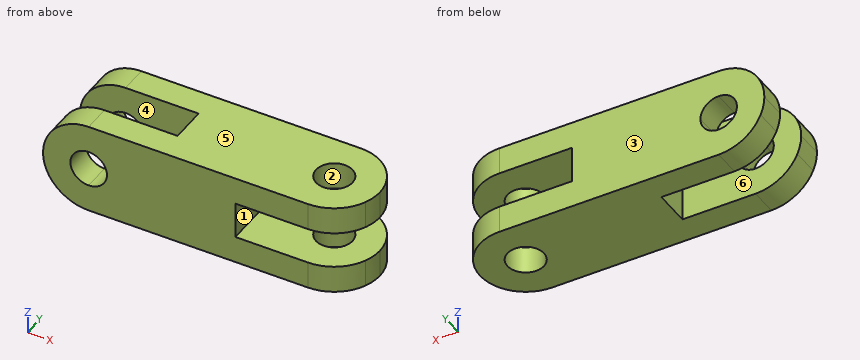
from build123d import *

# Parameters (mm, degrees)
F0_R     = 6.35
F1_DEPTH = 31.75
F0_W     = 41.275
F0_H     = 12.7
F3_DEPTH = 31.75
F2_W     = 41.275
F2_H     = 12.7
F4_DEPTH = 31.751
F5_DEPTH = 31.751


with BuildPart() as f1:
    # F0 (on Top) → F1 (new body)
    with BuildSketch(Plane.XY):
        with BuildLine():
            ThreePointArc((35.5833037704, -18.7424994532), (22.3013258492, -11.5625950536), (21.0336259389, 3.4825005468))
            Line((21.0336259389, 3.4825005468), (-15.2166962296, 3.4825005468))
            Line((-15.2166962296, 3.4825005468), (-15.2166962296, -9.2174994532))
            Line((-15.2166962296, -9.2174994532), (-56.4916962296, -9.2174994532))
            Line((-56.4916962296, -9.2174994532), (-56.4916962296, -18.7424994532))
            Line((-56.4916962296, -18.7424994532), (35.5833037704, -18.7424994532))
        make_face()
        with BuildLine():
            Line((35.5833037704, 13.0075005468), (-56.4916962296, 13.0075005468))
            Line((-56.4916962296, 13.0075005468), (-56.4916962296, 3.4825005468))
            Line((-56.4916962296, 3.4825005468), (-15.2166962296, 3.4825005468))
            Line((-15.2166962296, 3.4825005468), (21.0336259389, 3.4825005468))
            ThreePointArc((21.0336259389, 3.4825005468), (26.88820817, 10.414478468), (35.5833037704, 13.0075005468))
        make_face()
        with BuildLine():
            ThreePointArc((50.1329816019, 3.4825005468), (44.2783993708, 10.414478468), (35.5833037704, 13.0075005468))
            ThreePointArc((35.5833037704, 13.0075005468), (26.88820817, 10.414478468), (21.0336259389, 3.4825005468))
            ThreePointArc((21.0336259389, 3.4825005468), (22.3013258492, -11.5625950536), (35.5833037704, -18.7424994532))
            ThreePointArc((35.5833037704, -18.7424994532), (44.2783993708, -16.1494773745), (50.1329816019, -9.2174994532))
            ThreePointArc((50.1329816019, -9.2174994532), (51.1234414882, -6.1109150468), (51.4583037704, -2.8674994532))
            ThreePointArc((51.4583037704, -2.8674994532), (51.1234414882, 0.3759161403), (50.1329816019, 3.4825005468))
        make_face()
        with Locations((35.5833037704, -2.8674994532)):
            Circle(F0_R, mode=Mode.SUBTRACT)
        with BuildLine():
            ThreePointArc((50.1329816019, -9.2174994532), (44.2783993708, -16.1494773745), (35.5833037704, -18.7424994532))
            Line((35.5833037704, -18.7424994532), (51.6392476857, -18.7424994532))
            Line((51.6392476857, -18.7424994532), (51.4583037704, -9.2174994532))
            Line((51.4583037704, -9.2174994532), (50.1329816019, -9.2174994532))
        make_face()
        with BuildLine():
            Line((51.2197911739, 13.0075005468), (35.5833037704, 13.0075005468))
            ThreePointArc((35.5833037704, 13.0075005468), (44.2783993708, 10.414478468), (50.1329816019, 3.4825005468))
            Line((50.1329816019, 3.4825005468), (51.4583037704, 3.4825005468))
            Line((51.4583037704, 3.4825005468), (51.2197911739, 13.0075005468))
        make_face()
    extrude(amount=F1_DEPTH)

    # F0 (on Top) → F3 (cut)
    with BuildSketch(Plane.XY):
        with BuildLine():
            Line((35.5833037704, 13.0075005468), (-56.4916962296, 13.0075005468))
            Line((-56.4916962296, 13.0075005468), (-56.4916962296, 3.4825005468))
            Line((-56.4916962296, 3.4825005468), (-15.2166962296, 3.4825005468))
            Line((-15.2166962296, 3.4825005468), (21.0336259389, 3.4825005468))
            ThreePointArc((21.0336259389, 3.4825005468), (26.88820817, 10.414478468), (35.5833037704, 13.0075005468))
        make_face()
        with BuildLine():
            Line((51.2197911739, 13.0075005468), (35.5833037704, 13.0075005468))
            ThreePointArc((35.5833037704, 13.0075005468), (44.2783993708, 10.414478468), (50.1329816019, 3.4825005468))
            Line((50.1329816019, 3.4825005468), (51.4583037704, 3.4825005468))
            Line((51.4583037704, 3.4825005468), (51.2197911739, 13.0075005468))
        make_face()
        with BuildLine():
            ThreePointArc((50.1329816019, 3.4825005468), (44.2783993708, 10.414478468), (35.5833037704, 13.0075005468))
            ThreePointArc((35.5833037704, 13.0075005468), (26.88820817, 10.414478468), (21.0336259389, 3.4825005468))
            ThreePointArc((21.0336259389, 3.4825005468), (22.3013258492, -11.5625950536), (35.5833037704, -18.7424994532))
            ThreePointArc((35.5833037704, -18.7424994532), (44.2783993708, -16.1494773745), (50.1329816019, -9.2174994532))
            ThreePointArc((50.1329816019, -9.2174994532), (51.1234414882, -6.1109150468), (51.4583037704, -2.8674994532))
            ThreePointArc((51.4583037704, -2.8674994532), (51.1234414882, 0.3759161403), (50.1329816019, 3.4825005468))
        make_face()
        with Locations((35.5833037704, -2.8674994532)):
            Circle(F0_R, mode=Mode.SUBTRACT)
        with Locations((-35.8541962296, -2.8674994532)):
            Rectangle(F0_W, F0_H)
        with BuildLine():
            ThreePointArc((35.5833037704, -18.7424994532), (22.3013258492, -11.5625950536), (21.0336259389, 3.4825005468))
            Line((21.0336259389, 3.4825005468), (-15.2166962296, 3.4825005468))
            Line((-15.2166962296, 3.4825005468), (-15.2166962296, -9.2174994532))
            Line((-15.2166962296, -9.2174994532), (-56.4916962296, -9.2174994532))
            Line((-56.4916962296, -9.2174994532), (-56.4916962296, -18.7424994532))
            Line((-56.4916962296, -18.7424994532), (35.5833037704, -18.7424994532))
        make_face()
        with BuildLine():
            ThreePointArc((50.1329816019, -9.2174994532), (44.2783993708, -16.1494773745), (35.5833037704, -18.7424994532))
            Line((35.5833037704, -18.7424994532), (51.6392476857, -18.7424994532))
            Line((51.6392476857, -18.7424994532), (51.4583037704, -9.2174994532))
            Line((51.4583037704, -9.2174994532), (50.1329816019, -9.2174994532))
        make_face()
    extrude(amount=-F3_DEPTH, mode=Mode.SUBTRACT)

    # F2 (on face) → F4 (cut, through all)
    with BuildSketch(Plane.XZ.offset(18.7424994532)):
        with BuildLine():
            Line((-56.4916962296, 31.75), (-56.4916962296, 22.225))
            Line((-56.4916962296, 22.225), (-55.1663740611, 22.225))
            ThreePointArc((-55.1663740611, 22.225), (-49.31179183, 29.1569779212), (-40.6166962296, 31.75))
            Line((-40.6166962296, 31.75), (-56.4916962296, 31.75))
        make_face()
        with BuildLine():
            Line((-55.1663740611, 22.225), (-56.4916962296, 22.225))
            Line((-56.4916962296, 22.225), (-56.4916962296, 15.875))
            ThreePointArc((-56.4916962296, 15.875), (-56.1568339474, 19.1184155936), (-55.1663740611, 22.225))
        make_face()
        with BuildLine():
            ThreePointArc((-55.1663740611, 9.525), (-56.1568339474, 12.6315844064), (-56.4916962296, 15.875))
            Line((-56.4916962296, 15.875), (-56.4916962296, 9.525))
            Line((-56.4916962296, 9.525), (-55.1663740611, 9.525))
        make_face()
        with BuildLine():
            ThreePointArc((-40.6166962296, 0), (-49.31179183, 2.5930220788), (-55.1663740611, 9.525))
            Line((-55.1663740611, 9.525), (-56.4916962296, 9.525))
            Line((-56.4916962296, 9.525), (-56.4916962296, 0))
            Line((-56.4916962296, 0), (-40.6166962296, 0))
        make_face()
        with BuildLine():
            Line((-40.6166962296, 9.525), (-40.6166962296, 22.225))
            ThreePointArc((-40.6166962296, 22.225), (-46.9666962296, 15.875), (-40.6166962296, 9.525))
        make_face()
        with BuildLine():
            ThreePointArc((-34.2666962296, 15.875), (-36.126568169, 20.3651280605), (-40.6166962296, 22.225))
            Line((-40.6166962296, 22.225), (-40.6166962296, 9.525))
            ThreePointArc((-40.6166962296, 9.525), (-36.126568169, 11.3848719395), (-34.2666962296, 15.875))
        make_face()
        with Locations((31.0017476857, 15.875)):
            Rectangle(F2_W, F2_H)
    extrude(amount=-F4_DEPTH, mode=Mode.SUBTRACT)

    # F0 (on Top) → F5 (cut, through all)
    with BuildSketch(Plane.XY):
        with BuildLine():
            Line((51.2197911739, 13.0075005468), (35.5833037704, 13.0075005468))
            ThreePointArc((35.5833037704, 13.0075005468), (44.2783993708, 10.414478468), (50.1329816019, 3.4825005468))
            Line((50.1329816019, 3.4825005468), (51.4583037704, 3.4825005468))
            Line((51.4583037704, 3.4825005468), (51.2197911739, 13.0075005468))
        make_face()
        with BuildLine():
            ThreePointArc((50.1329816019, -9.2174994532), (44.2783993708, -16.1494773745), (35.5833037704, -18.7424994532))
            Line((35.5833037704, -18.7424994532), (51.6392476857, -18.7424994532))
            Line((51.6392476857, -18.7424994532), (51.4583037704, -9.2174994532))
            Line((51.4583037704, -9.2174994532), (50.1329816019, -9.2174994532))
        make_face()
    extrude(amount=F5_DEPTH, mode=Mode.SUBTRACT)


solid = f1.part
Geometry check sheet. Reference: the model listing, model coordinates, mm. Face numbers are marked on the shaded views. A direction names the side the tool comes from. Round coordinates to 2 decimals unless told otherwise and drop trailing zeros. Order: outer loops, then holes, each group sorted by start corner. A loop starts at its lowest first (then second) coordinate and runs counter-clockwise, first axis right, second up. Notation, with made-up numbers: M 13.25,-40 L 67.25,-40 A14 cw 67.25,-22 Z; hole C -35,62 d11. An arc over 180 degrees is marked long. Answer in a Markdown table with one row per item.
(1) Tool access check on the marked faces 1 and 2. Record the directions out of +Z, -Z, +X, -X, +Y, -Y that give a thin tool (end or side, any length) a straight path to the whole face; none if there is none.
Responses:
| item | result |
|---|---|
| face 1 | +X, +Y, -Y |
| face 2 | +Z, -Z |
(2) Scan lines: probe 1 along Z at (x, y) = (32.5, 7.5) (3 decimals); probe 2 along Y at (x, z) = (-47, 25); probe 3 along X at (y, z) = (2, 16). Record each from-to range of solid material in increasing order. Write a range as from..to.
Responses:
| item | result |
|---|---|
| probe 1 | z = 0..9.525, 22.225..31.75 |
| probe 2 | y = -18.74..-9.22, 3.48..13.01 |
| probe 3 | x = -15.22..10.36 |
(3) Go/stop test with flat-tipped pins: P1, Ø3, axis at y = -15, z = 22, coming from the +X side; P2, Ø10, axis at y = -3, z = 16.5, coming from the +X side; P3, Ø10, axis at y = -3, z = 15.5, coming from the -X side; P4, Ø1.5, axis at x = 39, y = 1.5, coming from the +Z side (3 decimals). Record where each tip stops, or that it passes through.
Responses:
| item | result |
|---|---|
| P1 | stops at x = 47.36 |
| P2 | stops at x = 10.36 |
| P3 | stops at x = -15.22 |
| P4 | passes through |
(4) Sectioned sample at B-B, the plane z = 21. Record the cut outline in (x, y), and give its area (3 significant figures).
Responses:
| item | result |
|---|---|
| outline | M -55.64,-18.74 L -44.37,-18.74 L -44.37,-9.22 L -55.64,-9.22 Z; M -55.64,3.48 L -44.37,3.48 L -44.37,13.01 L -55.64,13.01 Z; M -36.87,-18.74 L 10.36,-18.74 L 10.36,13.01 L -36.87,13.01 L -36.87,3.48 L -15.22,3.48 L -15.22,-9.22 L -36.87,-9.22 Z |
| area | 1,440 mm² |
(5) Sectioned sample at C-C, the plane y = 0.5. Record the cut outline in (x, z) (3 decimals), and give its area (3 significant figures).
Responses:
| item | result |
|---|---|
| outline | M -15.217,0 L 30.2,0 L 30.2,9.525 L 10.364,9.525 L 10.364,22.225 L 30.2,22.225 L 30.2,31.75 L -15.217,31.75 Z; M 40.967,0 L 51.097,0 L 51.097,9.525 L 40.967,9.525 Z; M 40.967,22.225 L 51.097,22.225 L 51.097,31.75 L 40.967,31.75 Z |
| area | 1,380 mm² |
(6) Sectioned sample at A-A, the plane x = -31.5. Record the cut outline in (y, z).
Responses:
| item | result |
|---|---|
| outline | M -18.74,0 L -9.22,0 L -9.22,31.75 L -18.74,31.75 Z; M 3.48,0 L 13.01,0 L 13.01,31.75 L 3.48,31.75 Z |
(7) Draft check along Y on the marked faces 3, 4, 5 and 6. Enter one of: released by +Y, released by -Y, zero draft, split by the parting line, or undercut.
Responses:
| item | result |
|---|---|
| face 3 | released by +Y |
| face 4 | undercut |
| face 5 | zero draft |
| face 6 | undercut |
